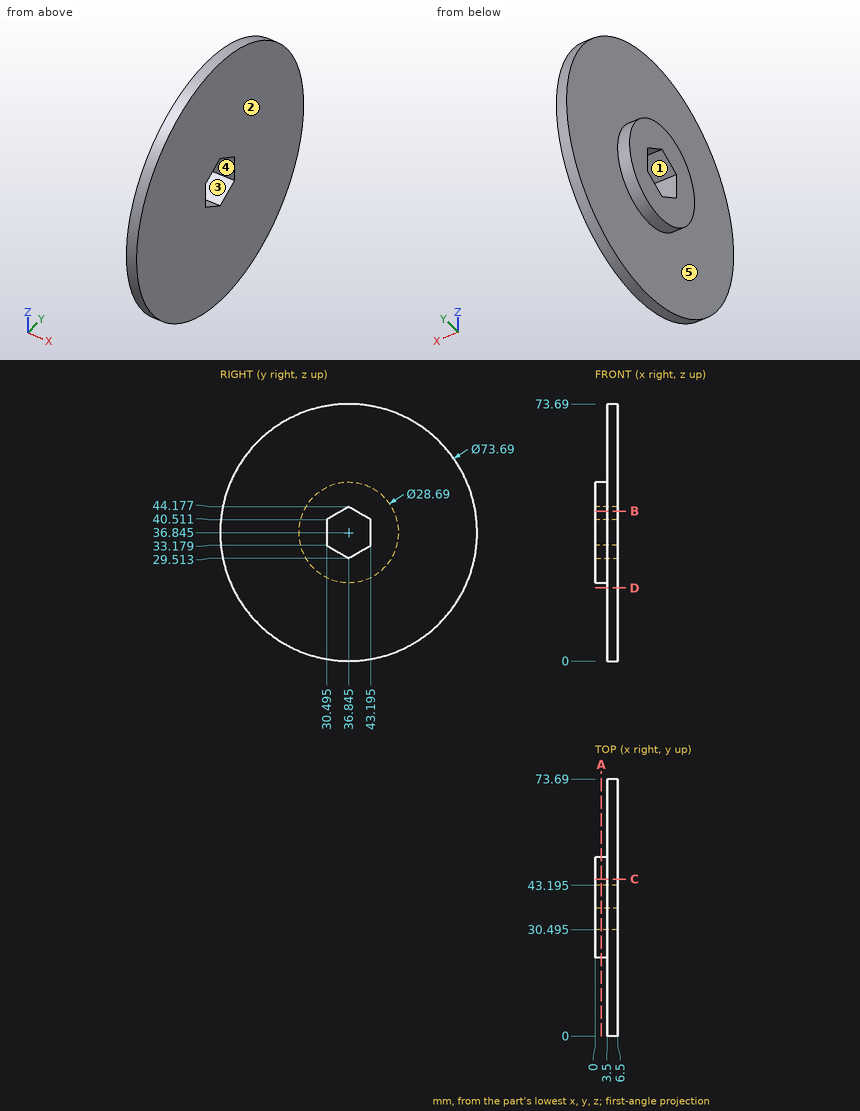
For this review, use the dimensioned drawing (mm, ordinates from the lowest corner) and the shaded views. A direction names the side the tool comes from. Round coordinates to 2 decimals unless told otherwise and drop trailing zeros. Order: outer loops, then holes, each group sorted by start corner. A loop starts at its lowest first (then second) coordinate and runs counter-clockwise, first axis right, second up. Notation, with made-up numbers: (21.25, 36.25) -> (29.25, 36.25) arc R14 cw to (29.25, 43.25) -> close; hole circle Ø5 at (-27.5, -5.5). An arc over 180 degrees is marked (long way). Put each result on its own line as item: value.
Q1. Machinability: for the marked faces 1 and 2, which of the approach directions +Z, -Z, +X, -X, +Y, -Y give a long, thin tool a straight path to every point of the face, cutting with its end or side? Answer none if there is none.
Check result:
face 1: +X, -X
face 2: +Z, -Z, +X, +Y, -Y
Q2. Insertion check: pin 1 Ø5 at (y, z) = (38.5, 11) entering from -X; pin 2 Ø3 at (x, z) = (2.5, 39.5) entering from -Y; pin 3 Ø3 at (x, z) = (4, 37) entering from +Y. Each pin has a flat end and moves straight along its axis. Give the tip position at first contact, or say it passes through.
Check result:
pin 1: x = 3.5
pin 2: y = 0.03
pin 3: y = 73.69
Q3. Add section C-C on y = 45. Write out the cut boundary in (x, z).
Check result:
outline: (0, 25.04) -> (3.5, 25.04) -> (3.5, 0.91) -> (6.5, 0.91) -> (6.5, 72.78) -> (3.5, 72.78) -> (3.5, 48.65) -> (0, 48.65) -> close
Q4. For probe 1 along X at (y, z) = (45, 12.5); probe 2 along Z at (x, y) = (0.5, 37.5) (1 decimal); probe 3 along Y at (x, z) = (1.5, 40.5) (1 decimal), list the stretches that pass through material, from the lowest coordinate up. Write a range as [from, to].
Check result:
probe 1: [3.5, 6.5]
probe 2: [22.5, 29.9], [43.8, 51.2]
probe 3: [23, 30.5], [43.2, 50.7]
Q5. Add section D-D on z = 21. Write out the cut boundary in (x, y).
Check result:
outline: (3.5, 3.58) -> (6.5, 3.58) -> (6.5, 70.11) -> (3.5, 70.11) -> close
Q6. Add section B-B on z = 43. Write out the cut boundary in (x, y), plus the area to 3 significant figures.
Check result:
outline: (0, 23.89) -> (3.5, 23.89) -> (3.5, 0.52) -> (6.5, 0.52) -> (6.5, 34.81) -> (0, 34.81) -> close; (0, 38.88) -> (6.5, 38.88) -> (6.5, 73.17) -> (3.5, 73.17) -> (3.5, 49.8) -> (0, 49.8) -> close
area: 282 mm2
Q7. Add section A-A on x = 1.75. Write out the cut boundary in (y, z) (1 decimal).
Check result:
outline: circle Ø28.7 at (36.8, 36.8); hole (30.5, 33.2) -> (36.8, 29.5) -> (43.2, 33.2) -> (43.2, 40.5) -> (36.8, 44.2) -> (30.5, 40.5) -> close
Q8. Mouldability with a two-part tool opening along Y and no side actions: class the marked faces 3, 4 and 5 as pulls with the +Y half, pulls with the -Y half, needs draft (parallel to the pull), parting line crosses it, or undercut.
Check result:
face 3: undercut
face 4: undercut
face 5: needs draft
